from build123d import *

# Parameters (mm, degrees)
F0_W      = 75
F0_H      = 75
F1_DEPTH  = 75
F2_SIZE   = 5
F3_DEPTH  = 5
F4_DEPTH  = 5
F5_DEPTH  = 5
F6_DEPTH  = 5
F7_DEPTH  = 5
F8_DEPTH  = 5
F9_DEPTH  = 5
F10_DEPTH = 5
F11_DEPTH = 5
F12_DEPTH = 5
F13_DEPTH = 5
F14_DEPTH = 5
F15_DEPTH = 25
F16_DEPTH = 25
F17_DEPTH = 25
F18_DEPTH = 25
F19_DEPTH = 25
F20_DEPTH = 25


with BuildPart() as f1:
    # F0 (on Top) → F1 (new body)
    with BuildSketch(Plane.XY):
        with Locations((-37.5, 37.5)):
            Rectangle(F0_W, F0_H)
    extrude(amount=F1_DEPTH)

    # F2
    f2_edges = [f1.edges().sort_by_distance(p)[0] for p in [
        (-75, 37.5, 75),
        (-37.5, 0, 75),
        (0, 37.5, 75),
        (-37.5, 75, 75),
        (0, 75, 37.5),
        (-75, 75, 37.5),
        (-37.5, 75, 0),
        (-75, 0, 37.5),
        (-75, 37.5, 0),
        (0, 37.5, 0),
        (0, 0, 37.5),
        (-37.5, 0, 0),
    ]]
    chamfer(f2_edges, length=F2_SIZE)

    # F3 (add): a face of the model
    f3_faces = [f1.faces().sort_by_distance(p)[0] for p in [
        (-72.5, 37.5, 72.5),
    ]]
    extrude(f3_faces, amount=F3_DEPTH)

    # F4 (add): a face of the model
    f4_faces = [f1.faces().sort_by_distance(p)[0] for p in [
        (-37.5, 72.5, 72.5),
    ]]
    extrude(f4_faces, amount=F4_DEPTH)

    # F5 (add): a face of the model
    f5_faces = [f1.faces().sort_by_distance(p)[0] for p in [
        (-2.5, 37.5, 72.5),
    ]]
    extrude(f5_faces, amount=F5_DEPTH)

    # F6 (add): a face of the model
    f6_faces = [f1.faces().sort_by_distance(p)[0] for p in [
        (-37.5, 2.5, 72.5),
    ]]
    extrude(f6_faces, amount=F6_DEPTH)

    # F7 (add): a face of the model
    f7_faces = [f1.faces().sort_by_distance(p)[0] for p in [
        (-2.5, 72.5, 37.5),
    ]]
    extrude(f7_faces, amount=F7_DEPTH)

    # F8 (add): a face of the model
    f8_faces = [f1.faces().sort_by_distance(p)[0] for p in [
        (-2.5, 37.5, 2.5),
    ]]
    extrude(f8_faces, amount=F8_DEPTH)

    # F9 (add): a face of the model
    f9_faces = [f1.faces().sort_by_distance(p)[0] for p in [
        (-2.5, 2.5, 37.5),
    ]]
    extrude(f9_faces, amount=F9_DEPTH)

    # F10 (add): a face of the model
    f10_faces = [f1.faces().sort_by_distance(p)[0] for p in [
        (-37.5, 72.5, 2.5),
    ]]
    extrude(f10_faces, amount=F10_DEPTH)

    # F11 (add): a face of the model
    f11_faces = [f1.faces().sort_by_distance(p)[0] for p in [
        (-37.5, 2.5, 2.5),
    ]]
    extrude(f11_faces, amount=F11_DEPTH)

    # F12 (add): a face of the model
    f12_faces = [f1.faces().sort_by_distance(p)[0] for p in [
        (-72.5, 72.5, 37.5),
    ]]
    extrude(f12_faces, amount=F12_DEPTH)

    # F13 (add): a face of the model
    f13_faces = [f1.faces().sort_by_distance(p)[0] for p in [
        (-72.5, 37.5, 2.5),
    ]]
    extrude(f13_faces, amount=F13_DEPTH)

    # F14 (add): a face of the model
    f14_faces = [f1.faces().sort_by_distance(p)[0] for p in [
        (-72.5, 2.5, 37.5),
    ]]
    extrude(f14_faces, amount=F14_DEPTH)

    # F15 (add): a face of the model
    f15_faces = [f1.faces().sort_by_distance(p)[0] for p in [
        (-75, 37.5, 37.5),
    ]]
    extrude(f15_faces, amount=F15_DEPTH)

    # F16 (add): a face of the model
    f16_faces = [f1.faces().sort_by_distance(p)[0] for p in [
        (-37.5, 37.5, 75),
    ]]
    extrude(f16_faces, amount=F16_DEPTH)

    # F17 (add): a face of the model
    f17_faces = [f1.faces().sort_by_distance(p)[0] for p in [
        (0, 37.5, 37.5),
    ]]
    extrude(f17_faces, amount=F17_DEPTH)

    # F18 (add): a face of the model
    f18_faces = [f1.faces().sort_by_distance(p)[0] for p in [
        (-37.5, 37.5, 0),
    ]]
    extrude(f18_faces, amount=F18_DEPTH)

    # F19 (add): a face of the model
    f19_faces = [f1.faces().sort_by_distance(p)[0] for p in [
        (-37.5, 0, 37.5),
    ]]
    extrude(f19_faces, amount=F19_DEPTH)

    # F20 (add): a face of the model
    f20_faces = [f1.faces().sort_by_distance(p)[0] for p in [
        (-37.5, 75, 37.5),
    ]]
    extrude(f20_faces, amount=F20_DEPTH)


solid = f1.part
Verification items for the finished model (mm, model axes). A direction names the side the tool comes from. Round coordinates to 2 decimals unless told otherwise and drop trailing zeros. Loops run counter-clockwise (first coordinate to the right, second up) from the corner with the lowest first, then second, coordinate; pieces in that order, holes last. Notation, with made-up numbers: (61, -33.75) - (103, -33.75) arc R33 ccw to (103, -0.75) - close; hole circle Ø2 at (79.25, -32.5). An arc over 180 degrees is marked (long way). Use one line per item in the form item = value.
1. Section check B-B on z = 36. Record the cut outline in (x, y), and give its area (3 significant figures).
A:
outline = (-100, 5) - (-75, 5) - (-78.54, 1.46) - (-73.54, -3.54) - (-70, 0) - (-70, -25) - (-5, -25) - (-5, 0) - (-1.46, -3.54) - (3.54, 1.46) - (0, 5) - (25, 5) - (25, 70) - (0, 70) - (3.54, 73.54) - (-1.46, 78.54) - (-5, 75) - (-5, 100) - (-70, 100) - (-70, 75) - (-73.54, 78.54) - (-78.54, 73.54) - (-75, 70) - (-100, 70) - close
area = 12,200 mm²
2. Access from +Z, -Z, +X, -X, +Y, -Y to the whole of each face (thin tool, end or side, straight path). Record for faces 5 (the flat face through (-37.96, 76, 76.07)), 6 (the flat face through (-5, 1, 1)), 7 (the flat face through (-5, 74, 1)).
A:
face_5 = +Z, +X, -X, +Y
face_6 = -Z, +X, -Y
face_7 = -Z, +X, +Y
3. Scan lines: probe 1 along X at (y, z) = (17, 76.5); probe 2 along Y at (x, z) = (-20, 79). Record each from-to range of solid material in increasing order.
A:
probe_1 = -75.57 to -71.5, -70 to -5, -3.5 to 0.57
probe_2 = 5 to 70
4. Draft check along X on faces 1 (the flat face through (-76, 37.04, 76.07)), 2 (the flat face through (-1, 74, 70)), 3 (the flat face through (-3, 37, -2)), 4 (the flat face through (-3, 77, 37)). Enter one of: pulls with the +X half, pulls with the -X half, needs draft (parallel to the pull), parting line crosses it, or undercut.
A:
face_1 = pulls with the -X half
face_2 = needs draft
face_3 = undercut
face_4 = undercut
5. Section check A-A on x = -10.5. Record the cut outline in (y, z).
A:
outline = (-25, 5) - (0, 5) - (-3.54, 1.46) - (1.46, -3.54) - (5, 0) - (5, -25) - (70, -25) - (70, 0) - (73.54, -3.54) - (78.54, 1.46) - (75, 5) - (100, 5) - (100, 70) - (75, 70) - (78.54, 73.54) - (73.54, 78.54) - (70, 75) - (70, 100) - (5, 100) - (5, 75) - (1.46, 78.54) - (-3.54, 73.54) - (0, 70) - (-25, 70) - close
6. Section check C-C on y = -9. Record the cut outline in (x, z), and give its area (4 significant figures).
A:
outline = (-70, 5) - (-5, 5) - (-5, 70) - (-70, 70) - close
area = 4,225 mm²
7. Gauge pin test, flat ends, axial feed: pin 1 Ø20 at (x, y) = (16, 53) entering from -Z; pin 2 Ø7.5 at (y, z) = (-12.5, 46) entering from +X; pin 3 Ø20 at (x, y) = (-47, 92) entering from +Z. Record the tip position at first contact, or that the pin passes through.
A:
pin_1 = 5
pin_2 = -5
pin_3 = 70
